```python
from build123d import *

# Parameters (mm, degrees)
F0_R     = 50
F1_DEPTH = 175
F5_D     = 90
F5_DEPTH = 175.001


with BuildPart() as f1:
    # F0 (on Front) → F1 (new body)
    with BuildSketch(Plane.XZ):
        Circle(F0_R)
    extrude(amount=F1_DEPTH)

    # F2 (on Front) → F3 (revolve)
    with BuildSketch(Plane.XZ):
        with BuildLine():
            Line((0, -49.6900500015), (0, 49.6900500015))
            ThreePointArc((0, 49.6900500015), (-49.6900500015, 0), (0, -49.6900500015))
        make_face()
    revolve(axis=Axis((0, 0, 0), (0, 0, -1)))

    # F5 (through all, one way)
    with BuildSketch(Plane(origin=(0, 0, 0), x_dir=(1, 0, 0), z_dir=(0, 1, 0))):
        with Locations((0, 0)):
            Circle(F5_D / 2)
    extrude(amount=-F5_DEPTH, mode=Mode.SUBTRACT)


solid = f1.part
```
The listing builds one solid part. Answer for the finished solid, in the listing's coordinates (mm). Coordinates: 2 decimals unless noted, no trailing zeros. Write each loop counter-clockwise with the first axis right and the second up, starting at its lowest first coordinate (ties: lowest second). Pieces come first, ordered by that corner, then holes. Notation, with made-up numbers: (74, -33.75) - (111, -33.75) arc R23 cw to (111, 1.25) - close; hole circle Ø9 at (2.25, 8.5). An arc over 180 degrees is marked (long way). Return JSON: item names as keys, results as strings. Group by question number.
1. Straight lines are drawn through the part: L1, parallel to Z at x = 0, y = -36; L2, parallel to X at y = -80, z = 13.5; L3, parallel to X at y = -164, z = -34.5. For each, find the intervals that lie inside material, in ascending order.
2. A cutting plane is placed at B-B, the plane x = 18.5. Determine the outline of the cut face in (y, z).
3. Determine the mould class of faces 1 (the cylindrical face through (47.69, -86.28, 15.02)), 2 (the flat face through (-41, -175, 19)), 3 (the cylindrical face through (20.765, -86.275, 39.923)) for opening direction Z: released by +Z, released by -Z, zero draft, split by the parting line, or undercut.
4. Given pin 1 (1.5 mm diameter, centred on x = -34, z = -28, fed in from +Y); pin 2 (5 mm diameter, centred on y = -10, z = -8, fed in from -X); pin 3 (12 mm diameter, centred on x = 12, y = -5.5, fed in from +Z), each flat-ended and moving along its own axis, determine where each tip first touches the part or whether it passes through.
5. A cutting plane is placed at C-C, the plane y = -84. Determine the outline of the cut face in (x, z).
6. A cutting plane is placed at A-A, the plane z = 0. Determine the outline of the cut face in (x, y).
Ans:
{
 "1": {"L1": "-50 to -45, 45 to 50", "L2": "-48.14 to -42.93, 42.93 to 48.14", "L3": "-36.19 to -28.89, 28.89 to 36.19"},
 "2": {"outline": "(-175, -46.45) - (0, -46.45) - (0, -46.12) arc R46.12 ccw to (0, 46.12) - (0, 46.45) - (-175, 46.45) - (-175, 41.02) - (0, 41.02) - (0, -41.02) - (-175, -41.02) - close"},
 "3": {"face 1": "split by the parting line", "face 2": "zero draft", "face 3": "undercut"},
 "4": {"pin 1": "y = 24.38", "pin 2": "x = -49.7", "pin 3": "z = 49.64"},
 "5": {"outline": "circle Ø100 at (0, 0); hole circle Ø90 at (0, 0)"},
 "6": {"outline": "(-50, -175) - (-45, -175) - (-45, 0) - (45, 0) - (45, -175) - (50, -175) - (50, 0) - (49.69, 0) arc R49.69 ccw to (-49.69, 0) - (-50, 0) - close"}
}
